from build123d import *

# Parameters (mm, degrees)
F0_W     = 20
F0_H     = 37.8
F0_W_2   = 7.15
F0_H_2   = 3.3
F0_W_3   = 7.5
F0_H_3   = 2.5
F1_DEPTH = 17
F3_DEPTH = 20.001
F4_R     = 2.3
F5_DEPTH = 17.001
F7_DEPTH = 5
F8_R     = 2.3
F9_DEPTH = 11


with BuildPart() as f1:
    # F0 (on Front) → F1 (new body)
    with BuildSketch(Plane.XZ):
        with Locations((0, 18.9)):
            Rectangle(F0_W, F0_H)
        with Locations((0, 6.65)):
            Rectangle(F0_W_2, F0_H_2, mode=Mode.SUBTRACT)
        with Locations((0, 11.55)):
            Rectangle(F0_W_3, F0_H_3, mode=Mode.SUBTRACT)
    extrude(amount=F1_DEPTH)

    # F2 (on face) → F3 (cut, through all)
    with BuildSketch(Plane.YZ.offset(10)):
        with BuildLine():
            Line((-9.75, 39.08921), (-9.75, 27.576743))
            ThreePointArc((-9.75, 27.576743), (-8.5, 14.9), (-7.25, 27.576743))
            Line((-7.25, 27.576743), (-7.25, 39.08921))
            Line((-7.25, 39.08921), (-9.75, 39.08921))
        make_face()
    extrude(amount=-F3_DEPTH, mode=Mode.SUBTRACT)

    # F4 (on face) → F5 (cut, through all)
    with BuildSketch(Plane(origin=(0, 0, 0), x_dir=(-1, 0, 0), z_dir=(0, 1, 0))):
        with Locations((0, 32.8)):
            Circle(F4_R)
    extrude(amount=-F5_DEPTH, mode=Mode.SUBTRACT)

    # F6 (on face) → F7 (cut)
    with BuildSketch(Plane(origin=(0, 0, 0), x_dir=(-1, 0, 0), z_dir=(0, 1, 0))):
        Polygon((4.128054, 32.8), (2.064027, 36.375), (-2.064027, 36.375), (-4.128054, 32.8), (-2.064027, 29.225), (2.064027, 29.225), align=None)
    extrude(amount=-F7_DEPTH, mode=Mode.SUBTRACT)

    # F8 (on face) → F9 (cut)
    with BuildSketch(Plane(origin=(0, 0, 0), x_dir=(1, 0, 0), z_dir=(0, 0, -1))):
        with Locations((0, 8.5)):
            Circle(F8_R)
    extrude(amount=-F9_DEPTH, mode=Mode.SUBTRACT)


solid = f1.part
CAD build for the part. Positions are in the model's coordinates, mm. A direction names the side the tool comes from. Round coordinates to 2 decimals unless told otherwise and drop trailing zeros. Write each loop counter-clockwise with the first axis right and the second up, starting at its lowest first coordinate (ties: lowest second). Pieces come first, ordered by that corner, then holes. Notation, with made-up numbers: M 24.25,46.5 L 83.25,46.5 A23 cw 83.25,80.5 Z; hole C -10.75,47 d1. An arc over 180 degrees is marked long. Put each result on its own line as item: value. Start each with the question number.
1) Saw through at D-D, the plane x = -5. Write the cut outline in (y, z).
2) Pull direction Y, two halves, no side cores. Call faces 1 (the flat face through (0, -17, 19)), 2 (the cylindrical face through (0.499, -6.109, 30.555)), 3 (the cylindrical face through (0.14, -8.764, 14.905)): pulls with the +Y half, pulls with the -Y half, needs draft (parallel to the pull), parting line crosses it, or undercut.
3) Pin check, flat tip, straight feed: pin 1 Ø2 at (x, y) = (0, -11) entering from -Z. Stop position of the tip, or through.
4) Saw through at C-C, the plane z = 9.5. Write the cut outline in (x, y).
5) Saw through at B-B, the plane y = -8.5. Write the cut outline in (x, z) (3 decimals), and give its area (3 significant figures).
6) Drill centre lines: probe 1 along Y at (x, z) = (0, 9.95); probe 2 along Z at (x, y) = (0, -13.5) (3 decimals); probe 3 along Y at (x, z) = (1.5, 35.5). Where is each one in solid material? Low to high. Write a range as [from, to].
7) 3-axis set-ups, long thin cutter, end or side, ignore diameter. For faces 4 (the flat face through (-3, -8, 10.3)), 5 (the flat face through (-3.11, -2.46, 34.56)), 6 (the flat face through (0, -9.75, 30)), 7 (the cylindrical face through (-0.3, -10.78, 2.46)): which of +Z, -Z, +X, -X, +Y, -Y reach the whole face in a straight line?
8) Saw through at A-A, the plane y = -15.5. Write the cut outline in (x, z) (3 decimals).
Resolved:
1. outline: M -17,0 L 0,0 L 0,37.8 L -7.25,37.8 L -7.25,27.58 A6.4 cw long -9.75,27.58 L -9.75,37.8 L -17,37.8 Z
2. face 1: pulls with the -Y half
2. face 2: needs draft
2. face 3: undercut
3. pin 1: z = 0
4. outline: M -10,-17 L 10,-17 L 10,0 L -10,0 Z; hole C 0,-8.5 d4.6
5. outline: M -10,0 L -2.3,0 L -2.3,5 L -3.575,5 L -3.575,8.3 L -2.3,8.3 L -2.3,10.3 L -3.75,10.3 L -3.75,12.8 L 3.75,12.8 L 3.75,10.3 L 2.3,10.3 L 2.3,8.3 L 3.575,8.3 L 3.575,5 L 2.3,5 L 2.3,0 L 10,0 L 10,14.9 L -10,14.9 Z
5. area: 223 mm²
6. probe 1: [-17, -10.8], [-6.2, 0]
6. probe 2: [0, 5], [8.3, 10.3], [12.8, 17.305], [25.295, 30.5], [35.1, 37.8]
6. probe 3: [-17, -9.75], [-7.25, -5]
7. face 4: +Y, -Y
7. face 5: +Y
7. face 6: +Z, +X, -X
7. face 7: -Z
8. outline: M -10,0 L 10,0 L 10,37.8 L -10,37.8 Z; hole M -3.75,10.3 L 3.75,10.3 L 3.75,12.8 L -3.75,12.8 Z; hole M -3.575,5 L 3.575,5 L 3.575,8.3 L -3.575,8.3 Z; hole C 0,32.8 d4.6
